Source: three-view drawing plus pictorial views. Frame: mm from the lowest corner of the part. A direction names the side the tool comes from. Give positions to 0.01 mm unless a question says otherwise; leave off trailing zeros. Order: outer loops, then holes, each group sorted by start corner. A loop starts at its lowest first (then second) coordinate and runs counter-clockwise, first axis right, second up. Notation, with made-up numbers: (-3, -7) -> (27, -7) arc R19 cw to (27, -3) -> close; hole circle Ø9 at (36.25, -15). An arc over 180 degrees is marked (long way). One line per question, with ' | ' between items.
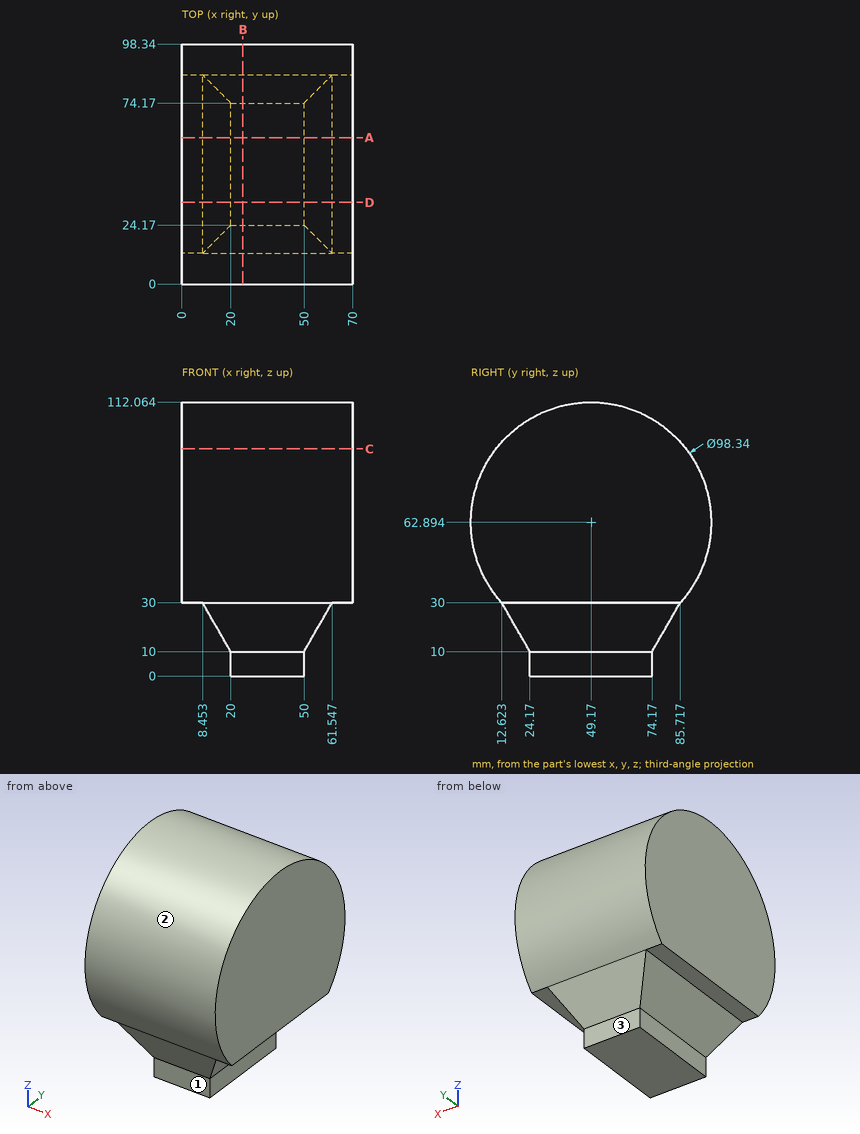
1) Section A-A on y = 60. Return loops of the section in (x, z), plus the area to 3 significant figures.
Check result:
outline: (0, 30) -> (8.45, 30) -> (20, 10) -> (20, 0) -> (50, 0) -> (50, 10) -> (61.55, 30) -> (70, 30) -> (70, 110.86) -> (0, 110.86) -> close | area: 6,790 mm^2
2) Contact query for flat-ended pins moving along their axis: pin 1 Ø4 at (x, y) = (5.5, 34) entering from -Z; pin 2 Ø1 at (x, z) = (52, 19) entering from -Y (3 decimals); pin 3 Ø3 at (x, y) = (37, 40) entering from +Z. Output: stop coordinate, or through.
Check result:
pin 1: stops at z = 30 | pin 2: stops at y = 18.685 | pin 3: stops at z = 111.46
3) Section C-C on z = 93. Return loops of the section in (x, y), plus the area to 3 significant figures.
Check result:
outline: (0, 10.29) -> (70, 10.29) -> (70, 88.05) -> (0, 88.05) -> close | area: 5,440 mm^2
4) Set-up query: the marked faces 1, 2 and 3. Return all of +Z, -Z, +X, -X, +Y, -Y with unobstructed straight access to the full face (end or side cutting, diameter ignored); none if empty.
Check result:
face 1: -Z, +X, -X, -Y | face 2: +X, -X | face 3: -Z, +X, -X, +Y
5) Material intervals for probe 1 along Z at (x, y) = (64.5, 48); probe 2 along Y at (x, z) = (21.5, 62); probe 3 along Y at (x, z) = (39, 93), sorted ascending. Write a range as from..to.
Check result:
probe 1: z = 30..112.05 | probe 2: y = 0.01..98.33 | probe 3: y = 10.29..88.05
6) Section B-B on x = 25. Return loops of the section in (y, z), plus the area to 3 significant figures.
Check result:
outline: (12.62, 30) -> (24.17, 10) -> (24.17, 0) -> (74.17, 0) -> (74.17, 10) -> (85.72, 30) arc R49.17 ccw (long way) to start | area: 8,500 mm^2
7) Section D-D on y = 33.5. Return loops of the section in (x, z), plus the area to 3 significant figures.
Check result:
outline: (0, 30) -> (8.45, 30) -> (20, 10) -> (20, 0) -> (50, 0) -> (50, 10) -> (61.55, 30) -> (70, 30) -> (70, 109.5) -> (0, 109.5) -> close | area: 6,700 mm^2
